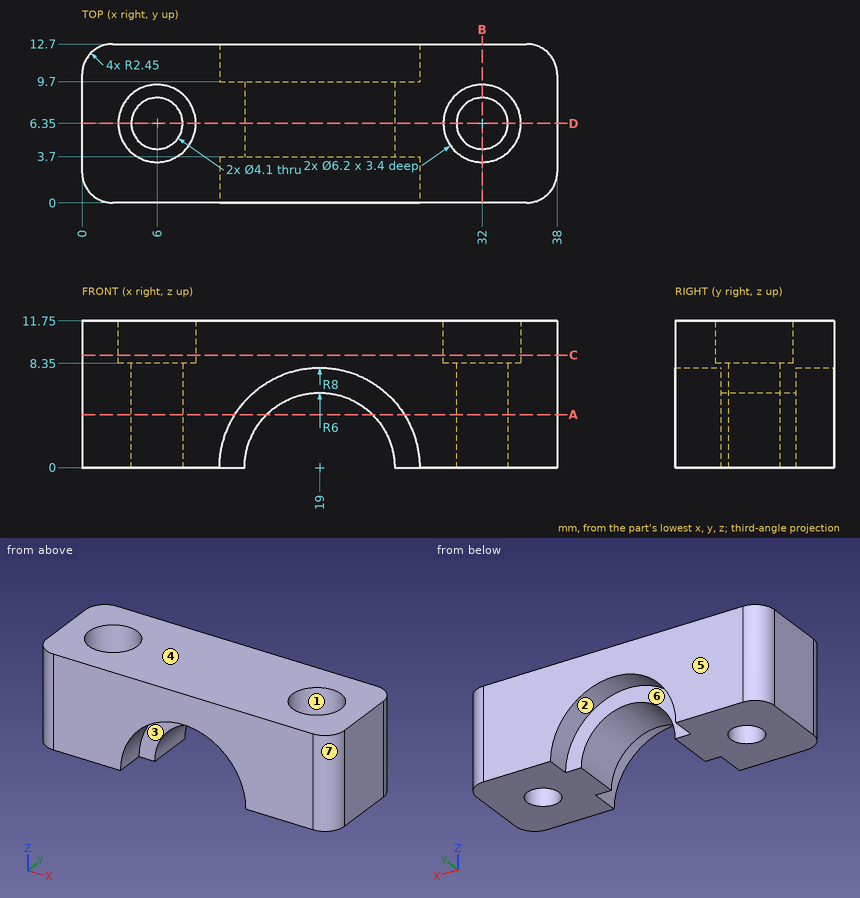
Job drawing, mm, ordinate dimensions from the low corner. One solid piece. A direction names the side the tool comes from. Coordinates: 2 decimals unless noted, no trailing zeros. Write each loop counter-clockwise with the first axis right and the second up, starting at its lowest first coordinate (ties: lowest second). Pieces come first, ordered by that corner, then holes. Notation, with made-up numbers: (41.5, -16) -> (46.5, -16) arc R27 ccw to (46.5, 4) -> close; hole circle Ø7 at (71, 58.25). An arc over 180 degrees is marked (long way). Use CSV: the item, a comma, the result in double quotes. Start each with the question number.
Item 1: Band-saw the part on A-A, the plane z = 4.25. Write the cut outline in (x, y), plus the area to 3 significant figures.
Item 2: Band-saw the part on C-C, the plane z = 9. Write the cut outline in (x, y), plus the area to 3 significant figures.
Item 3: Band-saw the part on D-D, the plane y = 6.35. Write the cut outline in (x, z), plus the area to 3 significant figures.
Item 4: Wall check: probe 1 along X at (y, z) = (4.5, 7); probe 2 along Y at (x, z) = (6, 6.5); probe 3 along X at (y, z) = (4.75, 8.75). Give the ranges that are in metal, low to high.
Item 5: Tool access for the marked faces 1, 2, 3 and 4: list every direction of +Z, -Z, +X, -X, +Y, -Y with a clear straight run to the whole face (end or side of a thin tool).
Item 6: Two-plate mould, pull along X, no slides. Class the marked faces 5, 6 and 7: +X half, -X half, draft (parallel to the pull), parting line (faces both ways), or undercut.
Item 7: Drop flat-ended pins along their axis: P1, Ø5.5, axis at x = 32, y = 6.35, coming from the +Z side; P2, Ø4, axis at x = 19, z = 5, coming from the -Y side; P3, Ø3, axis at x = 33.5, y = 7.5, coming from the +Z side; P4, Ø4, axis at x = 18.5, z = 5.5, coming from the +Y side. Give the stop position or say it passes through.
Item 8: Band-saw the part on B-B, the plane x = 32. Write the cut outline in (y, z), plus the area to 3 significant figures.
Response values:
1,outline,"(0, 2.45) arc R2.45 ccw to (2.45, 0) -> (12.22, 0) -> (12.22, 3.7) -> (14.76, 3.7) -> (14.76, 9.7) -> (12.22, 9.7) -> (12.22, 12.7) -> (2.45, 12.7) arc R2.45 ccw to (0, 10.25) -> close; (23.24, 3.7) -> (25.78, 3.7) -> (25.78, 0) -> (35.55, 0) arc R2.45 ccw to (38, 2.45) -> (38, 10.25) arc R2.45 ccw to (35.55, 12.7) -> (25.78, 12.7) -> (25.78, 9.7) -> (23.24, 9.7) -> close; hole circle Ø4.1 at (6, 6.35); hole circle Ø4.1 at (32, 6.35)"
1,area,"309 mm2"
2,outline,"(0, 2.45) arc R2.45 ccw to (2.45, 0) -> (35.55, 0) arc R2.45 ccw to (38, 2.45) -> (38, 10.25) arc R2.45 ccw to (35.55, 12.7) -> (2.45, 12.7) arc R2.45 ccw to (0, 10.25) -> close; hole circle Ø6.2 at (6, 6.35); hole circle Ø6.2 at (32, 6.35)"
2,area,"417 mm2"
3,outline,"(0, 0) -> (3.95, 0) -> (3.95, 8.35) -> (2.9, 8.35) -> (2.9, 11.75) -> (0, 11.75) -> close; (8.05, 0) -> (13, 0) arc R6 cw to (25, 0) -> (29.95, 0) -> (29.95, 8.35) -> (28.9, 8.35) -> (28.9, 11.75) -> (9.1, 11.75) -> (9.1, 8.35) -> (8.05, 8.35) -> close; (34.05, 0) -> (38, 0) -> (38, 11.75) -> (35.1, 11.75) -> (35.1, 8.35) -> (34.05, 8.35) -> close"
3,area,"279 mm2"
4,probe 1,"x = 0 to 5.12, 6.88 to 31.12, 32.88 to 38"
4,probe 2,"y = 0 to 4.3, 8.4 to 12.7"
4,probe 3,"x = 0 to 3.34, 8.66 to 29.34, 34.66 to 38"
5,face 1,"+Z"
5,face 2,"-Z, +Y"
5,face 3,"-Z, -Y"
5,face 4,"+Z, +X, -X, +Y, -Y"
6,face 5,"draft"
6,face 6,"undercut"
6,face 7,"+X half"
7,P1,"stops at z = 8.35"
7,P2,"stops at y = 3.7"
7,P3,"stops at z = 11.75"
7,P4,"stops at y = 9.7"
8,outline,"(0, 0) -> (4.3, 0) -> (4.3, 8.35) -> (3.25, 8.35) -> (3.25, 11.75) -> (0, 11.75) -> close; (8.4, 0) -> (12.7, 0) -> (12.7, 11.75) -> (9.45, 11.75) -> (9.45, 8.35) -> (8.4, 8.35) -> close"
8,area,"93.9 mm2"
